Source: CAD feature listing. Evaluate the final solid. Frame: model axes, mm. A direction names the side the tool comes from. Round coordinates to 2 decimals unless told otherwise and drop trailing zeros. Loops run counter-clockwise (first coordinate to the right, second up) from the corner with the lowest first, then second, coordinate; pieces in that order, holes last. Notation, with made-up numbers: (45, -5) -> (61, -5) arc R18 ccw to (61, 14) -> close; hole circle Ø7 at (31.5, 12.25). An arc over 180 degrees is marked (long way). Write item = value, one per line.
from build123d import *

# Parameters (mm, degrees)
BOSS_EXTRUDE1_START  = -0.50441
BOSS_EXTRUDE1_DEPTH  = 3
M3_CLEARANCE_HOLE1_D = 3.6
CHAMFER1_SIZE        = 20
CUT_EXTRUDE1_DEPTH   = 9
FILLET1_R            = 5
M3_CLEARANCE_HOLE2_D = 3.6


with BuildPart() as part:
    # Sketch3 → Boss-Extrude1 (new body)
    with BuildSketch(Plane(origin=(0, 0, -35.504410209), x_dir=(-1, 0, 0), z_dir=(0, 0, -1)).offset(BOSS_EXTRUDE1_START)):
        Polygon((-218.449999836, 74.7), (-263.37903282, 74.7), (-346.621494542, 177.349268983), (-294.797705634, 219.375284435), (-263.37903282, 180.63179067), (-233.345595882, 204.98712461), (-194.783185306, 157.434431261), (-224.816622244, 133.079097321), (-197.200065818, 99.024129816), (-218.449999836, 81.791695172), align=None)
    extrude(amount=BOSS_EXTRUDE1_DEPTH)

    # M3 Clearance Hole1 (through all)
    with Locations(Plane(origin=(0, 0, -38), x_dir=(-1, 0, 0), z_dir=(0, 0, -1))):
        with Locations((-264.683828169, 86.311168448), (-279.800535078, 104.952122614), (-321.371479078, 156.214746571), (-336.488185987, 174.855700737)):
            Hole(M3_CLEARANCE_HOLE1_D / 2)

    # Chamfer1
    chamfer1_edges = [part.edges().sort_by_distance(p)[0] for p in [
        (224.816622244, 133.079097321, -36.500000209),
        (263.37903282, 180.63179067, -36.500000209),
    ]]
    chamfer(chamfer1_edges, length=CHAMFER1_SIZE)

    # Sketch11 → Cut-Extrude1 (cut)
    with BuildSketch(Plane(origin=(0, 0, -38), x_dir=(-1, 0, 0), z_dir=(0, 0, -1))):
        Polygon((-211.265757933, 100.492566173), (-228.809311315, 122.126151879), (-251.146132676, 84.7), (-230.74013843, 84.7), align=None)
        Polygon((-254.500346294, 88.836201271), (-232.163524933, 126.26235315), (-273.396229931, 112.137393978), align=None)
        Polygon((-235.517738552, 130.39855442), (-254.413622188, 153.699747128), (-276.750443549, 116.273595249), align=None)
        Polygon((-280.104657167, 120.40979652), (-257.767835806, 157.835948399), (-299.000540804, 143.710989227), align=None)
        Polygon((-261.122049425, 161.972149669), (-280.017933061, 185.273342377), (-302.354754422, 147.847190498), align=None)
        Polygon((-305.708968041, 151.983391768), (-283.372146679, 189.409543648), (-324.604851677, 175.284584476), align=None)
        Polygon((-286.818200173, 193.658995967), (-296.266141991, 205.309592321), (-328.050905171, 179.534036795), align=None)
    extrude(amount=-CUT_EXTRUDE1_DEPTH, mode=Mode.SUBTRACT)

    # Fillet1
    fillet1_edges = [part.edges().sort_by_distance(p)[0] for p in [
        (218.449999836, 74.7, -36.500000209),
        (197.200065818, 99.024129816, -36.500000209),
        (194.783185306, 157.434431261, -36.500000209),
        (233.345595882, 204.98712461, -36.500000209),
        (294.797705634, 219.375284435, -36.500000209),
        (346.621494542, 177.349268983, -36.500000209),
        (263.37903282, 74.7, -36.500000209),
    ]]
    fillet(fillet1_edges, radius=FILLET1_R)

    # M3 Clearance Hole2 (through all)
    with Locations(Plane(origin=(0, 0, -38), x_dir=(-1, 0, 0), z_dir=(0, 0, -1))):
        with Locations((-209.81921101, 165.341079734), (-228.715065901, 188.642236994)):
            Hole(M3_CLEARANCE_HOLE2_D / 2)


solid = part.part
1. Set-up query: faces 4 (the face through (242.611, 197.473, -36.479)), 5 (the face through (219.88, 76.2, -36.52)), 6 (the face through (282.03, 154.81, -36.52)). Return all of +Z, -Z, +X, -X, +Y, -Y with unobstructed straight access to the full face (end or side cutting, diameter ignored); none if empty.
Evaluation:
face_4 = +Z, -Z, +Y
face_5 = +Z, -Z, -X, -Y
face_6 = +Z, -Z
2. Section query C-C (y = 170). Return the cut outline in (x, z).
Evaluation:
outline = (204.97, -38) -> (267.63, -38) -> (267.63, -35) -> (204.97, -35) -> close; (289.13, -38) -> (294.96, -38) -> (294.96, -35) -> (289.13, -35) -> close; (320.32, -38) -> (340.66, -38) -> (340.66, -35) -> (320.32, -35) -> close
3. Contact query for flat-ended pins moving along their axis: pin 1 Ø4 at (x, y) = (279.8, 104.95) entering from -Z; pin 2 Ø1 at (x, z) = (282.5, -35.5) entering from -Y; pin 3 Ø1.7 at (y, z) = (81, -37) entering from -X; pin 4 Ø1.5 at (y, z) = (147.5, -37.5) entering from +X. Output: stop coordinate, or through.
Evaluation:
pin_1 = -38
pin_2 = 97.66
pin_3 = 218.38
pin_4 = 323.02
4. Mould query, pull axis X, two halves, no side actions, for faces 1 (the face through (239.82, 103.68, -36.52)), 2 (the face through (303.6, 124.3, -36.5)), 3 (the face through (214.3, 181.5, -36.5)). Classes: released by +X, released by -X, zero draft, split by the parting line, or undercut.
Evaluation:
face_1 = undercut
face_2 = released by +X
face_3 = released by -X
5. Section query A-A (y = 110). Return the cut outline in (x, z).
Evaluation:
outline = (206.1, -38) -> (218.98, -38) -> (218.98, -35) -> (206.1, -35) -> close; (236.05, -38) -> (241.87, -38) -> (241.87, -35) -> (236.05, -35) -> close; (271.66, -38) -> (292.01, -38) -> (292.01, -35) -> (271.66, -35) -> close
6. Section query B-B (z = -35.75). Give the number of separate pieces and of enclosed holes in the cut face, then the cut area to 3 significant figures.
Evaluation:
separate_pieces = 1
enclosed_holes = 13
area = 8,620 mm²
7. Line query: probe 1 along X at (y, z) = (135.5, -35.9); probe 2 along Y at (x, z) = (250, -35.75); probe 3 along Y at (x, z) = (306.5, -37.9). Output: solid intervals per line, ascending. Write a range as from..to.
Evaluation:
probe_1 = 210.34..239.65, 265.28..271.1, 292.34..312.68
probe_2 = 74.7..84.7, 86.62..96.38, 120.15..125.44, 148.26..193.45
probe_3 = 127.87..152.96, 181.49..186.92, 197.01..209.89
